Here's how the part is built. I have some questions about the finished solid (model axes, mm). Face numbers are marked on the shaded views. A direction names the side the tool comes from. Coordinates: 2 decimals unless noted, no trailing zeros. Write each loop counter-clockwise with the first axis right and the second up, starting at its lowest first coordinate (ties: lowest second). Pieces come first, ordered by that corner, then holes.
Item 1: I want a section at B-B (z = 17.5). Please give me the cut outline in (x, y), and give its area (3 significant figures).
Item 2: I want a section at A-A (y = 0). Please give me the cut outline in (x, z).
Item 3: If we mould it in two halves opening along X, with no side actions, what happens to the marked faces 3, 4, 5 and 6? For each: pulls with the +X half, pulls with the -X half, needs draft (parallel to the pull), parting line crosses it, or undercut.
Item 4: I want a section at D-D (y = 8). Please give me the cut outline in (x, z), and give its area (3 significant figures).
Item 5: I want a section at C-C (x = 45). Please give me the cut outline in (y, z), and give its area (3 significant figures).
Item 6: I'm going to push flat-ended pins straight in: P1, Ø4, axis at x = 18.5, y = 5, coming from the +Z side; P2, Ø10, axis at y = -4, z = 12.5, coming from the +X side; P3, Ø4, axis at x = 46.5, z = 3, coming from the -Y side. Where does each tip first touch, or does it pass through?
Item 7: For the marked faces 1 and 2, which set-ups out of +Z, -Z, +X, -X, +Y, -Y let a thin tool reach every point of the face, with its end or its side?
Item 8: Please list where these lines run through material, in increasing order: line 1 (X direction, y = 6.5, z = 15.75); line 2 (X direction, y = 7, z = 3.75); line 3 (Y direction, x = 40.5, z = 8).
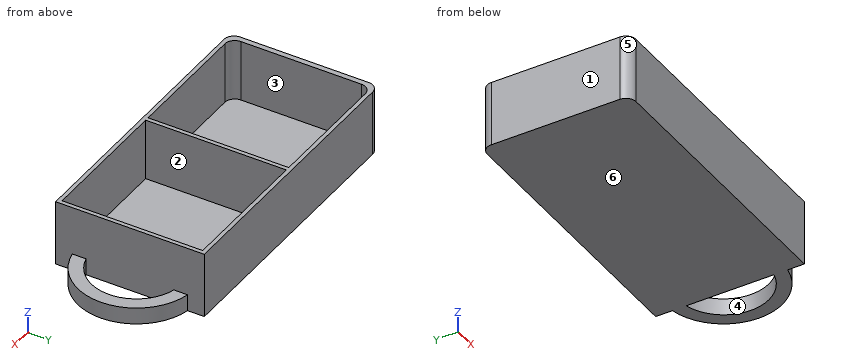
from build123d import *

# Parameters (mm, degrees)
SKETCH_1_W          = 86
SKETCH_1_H          = 44.4
EXTRUDE_1_DEPTH     = 19.6
EXTRUDE_2_DEPTH     = 5
SKETCH_3_W          = 40.8
SKETCH_3_H          = 42
SKETCH_3_W_2        = 41.2
CUT_EXTRUDE_1_DEPTH = 18.4
FILLET_1_R          = 3


with BuildPart() as part:
    # Эскиз1 → Бобышка-Вытянуть1 (new body)
    with BuildSketch(Plane.XY):
        Rectangle(SKETCH_1_W, SKETCH_1_H)
    extrude(amount=EXTRUDE_1_DEPTH)

    # Эскиз2 → Бобышка-Вытянуть2 (add)
    with BuildSketch(Plane.XY):
        with BuildLine():
            Line((43, 17.2), (43, 13.108775687))
            ThreePointArc((43, 13.108775687), (53.273546839, 0), (43, -13.108775687))
            Line((43, -13.108775687), (43, -17.2))
            ThreePointArc((43, -17.2), (57.273546839, 0), (43, 17.2))
        make_face()
    extrude(amount=EXTRUDE_2_DEPTH)

    # Эскиз3 → Вырез-Вытянуть1 (cut)
    with BuildSketch(Plane.XY.offset(19.6)):
        with Locations((-21, 0)):
            Rectangle(SKETCH_3_W, SKETCH_3_H)
        with Locations((21.2, 0)):
            Rectangle(SKETCH_3_W_2, SKETCH_3_H)
    extrude(amount=-CUT_EXTRUDE_1_DEPTH, mode=Mode.SUBTRACT)

    # Скругление1
    fillet_1_edges = [part.edges().sort_by_distance(p)[0] for p in [
        (-41.4, -21, 10.4),
        (-41.4, 21, 10.4),
        (-43, -22.2, 9.8),
        (-43, 22.2, 9.8),
    ]]
    fillet(fillet_1_edges, radius=FILLET_1_R)


solid = part.part
Answer:
1. outline: (-43, -19.2) arc R3 ccw to (-40, -22.2) - (43, -22.2) - (43, 22.2) - (-40, 22.2) arc R3 ccw to (-43, 19.2) - close; hole (-41.4, -18) arc R3 ccw to (-38.4, -21) - (-0.6, -21) - (-0.6, 21) - (-38.4, 21) arc R3 ccw to (-41.4, 18) - close; hole (0.6, -21) - (41.8, -21) - (41.8, 21) - (0.6, 21) - close
1. area: 374 mm2
2. outline: (-43, 0) - (43, 0) - (43, 19.6) - (41.8, 19.6) - (41.8, 1.2) - (0.6, 1.2) - (0.6, 19.6) - (-0.6, 19.6) - (-0.6, 1.2) - (-41.4, 1.2) - (-41.4, 19.6) - (-43, 19.6) - close; (53.27, 0) - (57.27, 0) - (57.27, 5) - (53.27, 5) - close
3. face 3: undercut
3. face 4: undercut
3. face 5: pulls with the -X half
3. face 6: needs draft
4. outline: (-43, 0) - (43, 0) - (43, 19.6) - (41.8, 19.6) - (41.8, 1.2) - (0.6, 1.2) - (0.6, 19.6) - (-0.6, 19.6) - (-0.6, 1.2) - (-41.4, 1.2) - (-41.4, 19.6) - (-43, 19.6) - close; (50.65, 0) - (55.34, 0) - (55.34, 5) - (50.65, 5) - close
4. area: 200 mm2
5. outline: (-16.7, 0) - (-12.45, 0) - (-12.45, 5) - (-16.7, 5) - close; (12.45, 0) - (16.7, 0) - (16.7, 5) - (12.45, 5) - close
5. area: 42.5 mm2
6. P1: stops at z = 1.2
6. P2: stops at x = 43
6. P3: stops at y = -16.85
7. face 1: +Z, -Z, -X, +Y, -Y
7. face 2: +Z
8. line 1: x = -43 to -41.4, -0.6 to 0.6, 41.8 to 43
8. line 2: x = -43 to -41.4, -0.6 to 0.6, 41.8 to 43, 51.32 to 55.81
8. line 3: y = -22.2 to -21, 21 to 22.2
